Work out the finished part from the listing and answer in its coordinate system (mm). Face numbers are marked on the shaded views. A direction names the side the tool comes from. Coordinates: 2 decimals unless noted, no trailing zeros. Order: outer loops, then holes, each group sorted by start corner. A loop starts at its lowest first (then second) coordinate and runs counter-clockwise, first axis right, second up. Notation, with made-up numbers: (37, 27.5) - (50, 27.5) arc R19 ccw to (50, 54.5) - close; hole circle Ø6 at (54, -19.5). An arc over 180 degrees is marked (long way). Use CSV: the item, a comma, the result in double quotes. Start each with the question number.
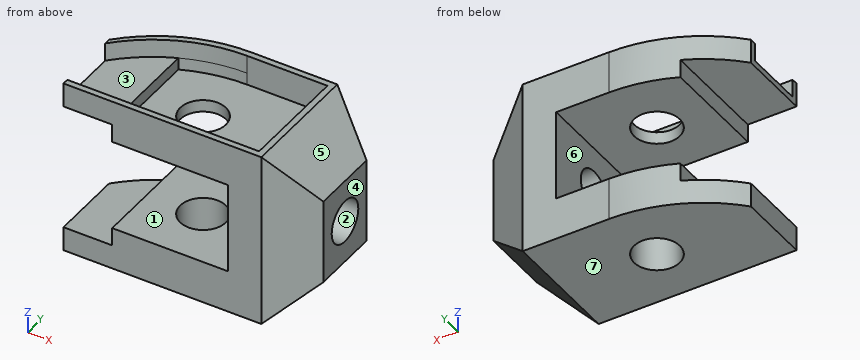
from build123d import *

# Parameters (mm, degrees)
SKETCH1_W           = 80
SKETCH1_H           = 58
BOSS_EXTRUDE1_DEPTH = 40
SKETCH2_R           = 7.5
CUT_EXTRUDE1_DEPTH  = 82.018516402
CUT_EXTRUDE6_DEPTH  = 64.568860301
SKETCH4_R           = 7
CUT_EXTRUDE7_DEPTH  = 95.026591983
CUT_EXTRUDE8_DEPTH  = 6
CUT_EXTRUDE9_DEPTH  = 4


with BuildPart() as part:
    # Sketch1 → Boss-Extrude1 (new body)
    with BuildSketch(Plane(origin=(0, 0, 0), x_dir=(1, 0, 0), z_dir=(0, 1, 0))):
        Rectangle(SKETCH1_W, SKETCH1_H)
    extrude(amount=BOSS_EXTRUDE1_DEPTH)

    # Sketch2 → Cut-Extrude1 (cut, through all)
    with BuildSketch(Plane.XY.offset(29)):
        Polygon((40, 40), (25, 40), (40, 31.339745962), align=None)
        with BuildLine():
            ThreePointArc((-40, 24), (-23.33939444, 35.82575695), (-3.33939444, 40))
            Line((-3.33939444, 40), (-40, 40))
            Line((-40, 40), (-40, 24))
        make_face()
        Polygon((40, 0), (40, 8.660254038), (25, 0), align=None)
        with Locations((-6, 19)):
            Circle(SKETCH2_R)
    extrude(amount=-CUT_EXTRUDE1_DEPTH, mode=Mode.SUBTRACT)

    # Sketch3 → Cut-Extrude6 (cut, through all)
    with BuildSketch(Plane(origin=(0, 0, 0), x_dir=(1, 0, 0), z_dir=(0, 1, 0))):
        Polygon((25, 29), (40, 29), (40, 14), align=None)
        Polygon((40, -14), (25, -29), (40, -29), align=None)
        Polygon((-40, 21), (-24, 21), (-24, 15), (14, 15), (14, -15), (-24, -15), (-24, -21), (-40, -21), align=None)
    extrude(amount=CUT_EXTRUDE6_DEPTH, mode=Mode.SUBTRACT)

    # Sketch4 → Cut-Extrude7 (cut, through all)
    with BuildSketch(Plane(origin=(40, 0, 0), x_dir=(0, 0, -1), z_dir=(1, 0, 0))):
        with Locations((0, 20)):
            Circle(SKETCH4_R)
    extrude(amount=-CUT_EXTRUDE7_DEPTH, mode=Mode.SUBTRACT)

    # Sketch5 → Cut-Extrude8 (cut)
    with BuildSketch(Plane.XY.offset(29)):
        with BuildLine():
            Line((-40, 2), (23, 2))
            Line((23, 2), (23, 38))
            Line((23, 38), (-3.33939444, 38))
            ThreePointArc((-3.33939444, 38), (-23.33939444, 33.82575695), (-40, 22))
            Line((-40, 22), (-40, 2))
        make_face()
    extrude(amount=-CUT_EXTRUDE8_DEPTH, mode=Mode.SUBTRACT)

    # Sketch6 → Cut-Extrude9 (cut)
    with BuildSketch(Plane.XY.offset(23)):
        with BuildLine():
            Line((-23.33939444, 33.82575695), (-23.33939444, 2))
            Line((-23.33939444, 2), (23, 2))
            Line((23, 2), (23, 38))
            Line((23, 38), (-3.33939444, 38))
            ThreePointArc((-3.33939444, 38), (-13.554876625, 36.945315647), (-23.33939444, 33.82575695))
        make_face()
    extrude(amount=-CUT_EXTRUDE9_DEPTH, mode=Mode.SUBTRACT)


solid = part.part
1) Flat-ended cylindrical pins translate along their axes: P1, Ø1.8, axis at y = 25, z = 16.5, coming from the -X side; P2, Ø4.5, axis at y = 12, z = 22, coming from the +X side; P3, Ø8, axis at y = 34, z = 20.5, coming from the +X side. Find the tip coordinate at first contact, or state that the pin passes through.
2) For a pull along Z with two mould halves and no side action, classify the marked faces 4, 5, 6 and 7 as +Z half, -Z half, draft (parallel to the pull), parting line (faces both ways), or undercut.
3) The part is cut by section C-C on x = -31. Determine the outline of the cut face in (y, z), plus the area to 3 significant figures.
4) The part is cut by section A-A on z = 0. Determine the outline of the cut face in (x, y), plus the area to 3 significant figures.
5) Straight lines are drawn through the part: line 1 (Z direction, x = -14.5, y = 37); line 2 (Z direction, x = -8, y = 32); line 3 (X direction, y = 23.5, z = -17). For each, find the intervals that lie inside material, in ascending order. Write a range as [from, to].
6) The part is cut by section B-B on y = 23. State how many separate pieces and enclosed holes the cut face has, plus the area to 3 significant figures.
7) The part is cut by section D-D on x = -6. Determine the outline of the cut face in (y, z).
8) For the marked faces 1, 2 and 3, determine the directions among +Z, -Z, +X, -X, +Y, -Y from which every point of the face is accessible in a straight line to the end or side of a thin tool.
Answer key:
1,P1,"x = -24"
1,P2,"x = 34.25"
1,P3,"x = 37.34"
2,face 4,"draft"
2,face 5,"+Z half"
2,face 6,"undercut"
2,face 7,"-Z half"
3,outline,"(0, -29) - (31.65, -29) - (31.65, -21) - (0, -21) - close; (0, 21) - (31.65, 21) - (31.65, 29) - (29.65, 29) - (29.65, 23) - (2, 23) - (2, 29) - (0, 29) - close"
3,area,"341 mm^2"
4,outline,"(14, 0) - (25, 0) - (40, 8.66) - (40, 13) - (14, 13) - close; (14, 27) - (40, 27) - (40, 31.34) - (25, 40) - (14, 40) - close"
4,area,"546 mm^2"
5,line 1,"[-29, -15], [15, 29]"
5,line 2,"[-29, -15], [15, 19]"
5,line 3,"[-24, -12], [0, 37]"
6,separate pieces,"4"
6,enclosed holes,"0"
6,area,"1,490 mm^2"
7,outline,"(0, -29) - (11.5, -29) - (11.5, -15) - (0, -15) - close; (0, 15) - (11.5, 15) - (11.5, 19) - (2, 19) - (2, 29) - (0, 29) - close; (26.5, -29) - (39.93, -29) - (39.93, -15) - (26.5, -15) - close; (26.5, 15) - (39.93, 15) - (39.93, 29) - (37.93, 29) - (37.93, 19) - (26.5, 19) - close"
8,face 1,"-X, +Y, -Y"
8,face 2,"+X, -X"
8,face 3,"+Z"
